```python
from build123d import *

# Parameters (mm, degrees)
SKETCH1_W           = 82.55
SKETCH1_H           = 57.15
BOSS_EXTRUDE2_DEPTH = 5.715
SKETCH1_7_W         = 88.9
SKETCH1_7_H         = 63.5
SKETCH1_7_W_2       = 82.55
SKETCH1_7_H_2       = 57.15
TOP_DEPTH           = 2.54
FRONTLIP_DEPTH      = 3.175
SKETCH4_R           = 1.5
M3SCREWHOLE_DEPTH   = 13.208
FILLET1_R           = 2.54
SKETCH5_R           = 3.5
SCREWHEADHOLE_DEPTH = 3.175


with BuildPart() as part:
    # Sketch1 → Boss-Extrude2 (new body)
    with BuildSketch(Plane(origin=(0, 0, 0), x_dir=(1, 0, 0), z_dir=(0, 1, 0))):
        Rectangle(SKETCH1_W, SKETCH1_H)
    extrude(amount=BOSS_EXTRUDE2_DEPTH)

    # Sketch1<7> → Top (add)
    with BuildSketch(Plane(origin=(0, 0, 0), x_dir=(1, 0, 0), z_dir=(0, 1, 0))):
        Rectangle(SKETCH1_7_W, SKETCH1_7_H)
        Rectangle(SKETCH1_7_W_2, SKETCH1_7_H_2, mode=Mode.SUBTRACT)
    extrude(amount=TOP_DEPTH)

    # Sketch3 → FrontLip (add)
    with BuildSketch(Plane.ZY.offset(44.45)):
        Polygon((-28.575, 2.54), (28.575, 2.54), (28.575, 13.97), (5.08, 13.97), (5.08, 11.43), (-5.08, 11.43), (-5.08, 13.97), (-28.575, 13.97), align=None)
    extrude(amount=-FRONTLIP_DEPTH)

    # Sketch4 → M3ScrewHole (cut)
    with BuildSketch(Plane(origin=(0, 5.715, 0), x_dir=(1, 0, 0), z_dir=(0, 1, 0))):
        with Locations(Location((-36.195, 23.495, 0), (0, 0, 270))):
            Circle(SKETCH4_R)
        with Locations(Location((36.195, 23.495, 0), (0, 0, 270))):
            Circle(SKETCH4_R)
        with Locations(Location((36.195, -23.495, 0), (0, 0, 270))):
            Circle(SKETCH4_R)
        with Locations(Location((-36.195, -23.495, 0), (0, 0, 270))):
            Circle(SKETCH4_R)
    extrude(amount=-M3SCREWHOLE_DEPTH, mode=Mode.SUBTRACT)

    # Fillet1
    fillet1_edges = [part.edges().sort_by_distance(p)[0] for p in [
        (-42.8625, 11.43, -5.08),
        (-42.8625, 11.43, 5.08),
        (44.45, 1.27, 31.75),
        (44.45, 1.27, -31.75),
        (-44.45, 1.27, 31.75),
        (-44.45, 1.27, -31.75),
    ]]
    fillet(fillet1_edges, radius=FILLET1_R - 0.0001)  # a hair under: the kernel refuses the full size

    # Sketch5 → ScrewHeadHole (cut)
    with BuildSketch(Plane.XZ):
        with Locations(Location((-36.195, 23.495, 0), (0, 0, 270))):
            Circle(SKETCH5_R)
        with Locations(Location((-36.195, -23.495, 0), (0, 0, 270))):
            Circle(SKETCH5_R)
        with Locations(Location((36.195, -23.495, 0), (0, 0, 270))):
            Circle(SKETCH5_R)
        with Locations(Location((36.195, 23.495, 0), (0, 0, 270))):
            Circle(SKETCH5_R)
    extrude(amount=-SCREWHEADHOLE_DEPTH, mode=Mode.SUBTRACT)


solid = part.part
```
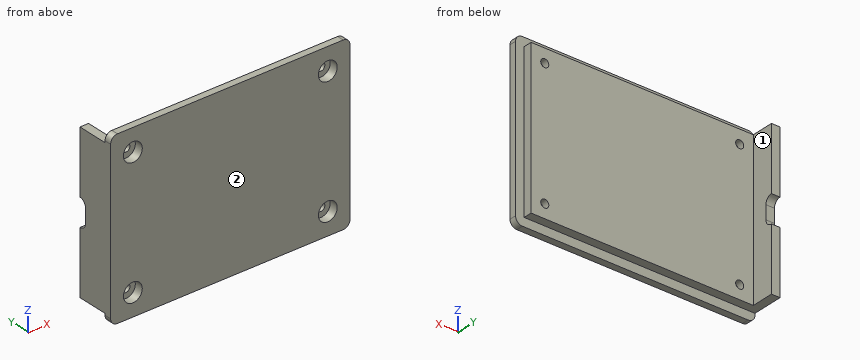
Work out the finished part from the listing and answer in its coordinate system (mm). Face numbers are marked on the shaded views. A direction names the side the tool comes from. Round coordinates to 2 decimals unless told otherwise and drop trailing zeros. Order: outer loops, then holes, each group sorted by start corner. A loop starts at its lowest first (then second) coordinate and runs counter-clockwise, first axis right, second up.
Q1. A tool of negligible diameter and unlimited length cuts with its end or side. For the marked faces 1 and 2, from which of +Z, -Z, +X, -X, +Y, -Y can it reach the whole face along a straight path? Write none if from no direction.
Solution:
face 1: +Z, -Z, +X, +Y
face 2: +Z, -Z, +X, -X, -Y
Q2. A cutting plane is placed at D-D, the plane z = 6. Determine the outline of the cut face in (x, y) (3 decimals).
Solution:
outline: (-44.45, 0) - (44.45, 0) - (44.45, 2.54) - (41.275, 2.54) - (41.275, 5.715) - (-41.275, 5.715) - (-41.275, 13.97) - (-44.45, 13.97) - close
Q3. A cutting plane is placed at B-B, the plane x = 1.5. Determine the outline of the cut face in (y, z) (3 decimals), then the cut area to 3 significant figures.
Solution:
outline: (0, -31.75) - (2.54, -31.75) - (2.54, -28.575) - (5.715, -28.575) - (5.715, 28.575) - (2.54, 28.575) - (2.54, 31.75) - (0, 31.75) - close
area: 343 mm2
Q4. A cutting plane is placed at A-A, the plane z = -23.5. Determine the outline of the cut face in (x, y) (3 decimals).
Solution:
outline: (-44.45, 0) - (-39.695, 0) - (-39.695, 3.175) - (-37.695, 3.175) - (-37.695, 5.715) - (-41.275, 5.715) - (-41.275, 13.97) - (-44.45, 13.97) - close; (-34.695, 3.175) - (-32.695, 3.175) - (-32.695, 0) - (32.695, 0) - (32.695, 3.175) - (34.695, 3.175) - (34.695, 5.715) - (-34.695, 5.715) - close; (37.695, 3.175) - (39.695, 3.175) - (39.695, 0) - (44.45, 0) - (44.45, 2.54) - (41.275, 2.54) - (41.275, 5.715) - (37.695, 5.715) - close
Q5. A cutting plane is placed at C-C, the plane y = 12.5. Determine the outline of the cut face in (x, z) (3 decimals), then the cut area to 3 significant figures.
Solution:
outline: (-44.45, -28.575) - (-41.275, -28.575) - (-41.275, -4.611) - (-44.45, -4.611) - close; (-44.45, 4.611) - (-41.275, 4.611) - (-41.275, 28.575) - (-44.45, 28.575) - close
area: 152 mm2
Q6. Find the intervals of material crossed by line 1 along X through (y, z) = (3, -21) (3 decimals); line 2 along Y through (x, z) = (29, -2) (3 decimals); line 3 along X through (y, z) = (5, 3.5) (3 decimals), in increasing order.
Solution:
line 1: x = -44.45 to -38.65, -33.74 to 33.74, 38.65 to 41.275
line 2: y = 0 to 5.715
line 3: x = -44.45 to 41.275
Q7. Given pin 1 Ø3.5 at (x, z) = (-36.195, 23.495) entering from -Y (3 decimals); pin 2 Ø5.5 at (x, z) = (-34.5, 24.5) entering from -Y; pin 3 Ø6 at (y, z) = (6, -18.5) entering from +X (3 decimals); pin 4 Ø17 at (x, z) = (3.5, -8.5) entering from +Y (3 decimals), each flat-ended and moving along its own axis, determine where each tip first touches the part or whether it passes through.
Solution:
pin 1: stops at y = 3.175
pin 2: stops at y = 0
pin 3: stops at x = 41.275
pin 4: stops at y = 5.715
